```python
from build123d import *

# Parameters (mm, degrees)
ESQUISSE1_W             = 76
ESQUISSE1_H             = 76
ESQUISSE1_W_2           = 70
ESQUISSE1_H_2           = 70
BOSS_EXTRU_2_DEPTH      = 101
ESQUISSE2_W             = 76
ESQUISSE2_H             = 76
BOSS_EXTRU_3_DEPTH      = 5
ESQUISSE3_W             = 76
ESQUISSE3_H             = 76
BOSS_EXTRU_4_DEPTH      = 5
ESQUISSE4_W             = 60
ESQUISSE4_H             = 44.878799425
ESQUISSE4_H_2           = 41.121200575
ENL_V_MAT_EXTRU_1_DEPTH = 80
ESQUISSE5_W             = 43.832159463
ESQUISSE5_H             = 60
ESQUISSE5_W_2           = 42.167840537
ENL_V_MAT_EXTRU_2_DEPTH = 80
ESQUISSE8_W             = 15
ESQUISSE8_H             = 30
BOSS_EXTRU_6_DEPTH      = 50
CONG_6_R                = 10
CONG_7_R                = 10
ESQUISSE10_R            = 5.5
ENL_V_MAT_EXTRU_3_DEPTH = 25
ESQUISSE11_R            = 7.5
ENL_V_MAT_EXTRU_4_DEPTH = 1


with BuildPart() as part:
    # Esquisse1 → Boss.-Extru.2 (new body)
    with BuildSketch(Plane.XY):
        with Locations((1.043095631, -5.469290785)):
            Rectangle(ESQUISSE1_W, ESQUISSE1_H)
        with Locations((1.043095631, -5.469290785)):
            Rectangle(ESQUISSE1_W_2, ESQUISSE1_H_2, mode=Mode.SUBTRACT)
    extrude(amount=BOSS_EXTRU_2_DEPTH)

    # Esquisse2 → Boss.-Extru.3 (add)
    with BuildSketch(Plane.XY.offset(101)):
        with Locations((1.043095631, -5.469290785)):
            Rectangle(ESQUISSE2_W, ESQUISSE2_H)
    extrude(amount=BOSS_EXTRU_3_DEPTH)

    # Esquisse3 → Boss.-Extru.4 (add)
    with BuildSketch(Plane(origin=(0, 0, 0), x_dir=(-1, 0, 0), z_dir=(0, 0, -1))):
        with Locations((-1.043095631, -5.469290785)):
            Rectangle(ESQUISSE3_W, ESQUISSE3_H)
    extrude(amount=BOSS_EXTRU_4_DEPTH)

    # Esquisse4 → Enlèv. mat.-Extru.1 (cut)
    with BuildSketch(Plane(origin=(0, 32.530709215, 0), x_dir=(1, 0, 0), z_dir=(0, 1, 0))):
        with Locations((1.043095631, -27.439399713)):
            Rectangle(ESQUISSE4_W, ESQUISSE4_H)
        with Locations((1.043095631, -75.439399713)):
            Rectangle(ESQUISSE4_W, ESQUISSE4_H_2)
    extrude(amount=-ENL_V_MAT_EXTRU_1_DEPTH, mode=Mode.SUBTRACT)

    # Esquisse5 → Enlèv. mat.-Extru.2 (cut)
    with BuildSketch(Plane.ZY.offset(36.956904369)):
        with Locations((26.916079732, -5.469290785)):
            Rectangle(ESQUISSE5_W, ESQUISSE5_H)
        with Locations((74.916079732, -5.469290785)):
            Rectangle(ESQUISSE5_W_2, ESQUISSE5_H)
    extrude(amount=-ENL_V_MAT_EXTRU_2_DEPTH, mode=Mode.SUBTRACT)

    # Esquisse8 → Boss.-Extru.6 (add)
    with BuildSketch(Plane.XY.offset(106)):
        with Locations((1.043095631, -5.469290785)):
            Rectangle(ESQUISSE8_W, ESQUISSE8_H)
    extrude(amount=BOSS_EXTRU_6_DEPTH)

    # Congé6
    cong_6_edges = [part.edges().sort_by_distance(p)[0] for p in [
        (1.043095631, -20.469290785, 156),
    ]]
    fillet(cong_6_edges, radius=CONG_6_R)

    # Congé7
    cong_7_edges = [part.edges().sort_by_distance(p)[0] for p in [
        (1.043095631, 9.530709215, 156),
    ]]
    fillet(cong_7_edges, radius=CONG_7_R)

    # Esquisse10 → Enlèv. mat.-Extru.3 (cut)
    with BuildSketch(Plane.ZY.offset(6.456904369)):
        with Locations(Location((141, -5.469290785, 0), (0, 0, 270))):
            Circle(ESQUISSE10_R)
    extrude(amount=-ENL_V_MAT_EXTRU_3_DEPTH, mode=Mode.SUBTRACT)

    # Esquisse11 → Enlèv. mat.-Extru.4 (cut)
    with BuildSketch(Plane.ZY.offset(6.456904369)):
        with Locations(Location((141, -5.469290785, 0), (0, 0, 270))):
            Circle(ESQUISSE11_R)
    extrude(amount=-ENL_V_MAT_EXTRU_4_DEPTH, mode=Mode.SUBTRACT)


solid = part.part
```
Read the model definition and answer for the solid it produces. Units are mm, in the model's axes. A direction names the side the tool comes from. Coordinates: 2 decimals unless noted, no trailing zeros. Write each loop counter-clockwise with the first axis right and the second up, starting at its lowest first coordinate (ties: lowest second). Pieces come first, ordered by that corner, then holes. Notation, with made-up numbers: (20, 71.25) -> (68, 71.25) arc R23 cw to (68, 107.25) -> close; hole circle Ø10 at (-2.75, -10). An arc over 180 degrees is marked (long way). Return JSON: item names as keys, results as strings.
1. A cutting plane is placed at C-C (z = 141). Determine the outline of the cut face in (x, y), and give its area (3 significant figures).
Found:
{"outline": "(-6.46, -20.47) -> (8.54, -20.47) -> (8.54, -10.97) -> (-5.46, -10.97) -> (-5.46, -12.97) -> (-6.46, -12.97) -> close; (-6.46, 2.03) -> (-5.46, 2.03) -> (-5.46, 0.03) -> (8.54, 0.03) -> (8.54, 9.53) -> (-6.46, 9.53) -> close", "area": "281 mm2"}
2. A tool of negligible diameter and unlimited length cuts with its end or side. For faces 4 (the face through (1, 31, 5)), 5 (the face through (-35, 24.531, 27)), 6 (the face through (1, 9.531, 126)), from which of +Z, -Z, +X, -X, +Y, -Y can it reach the whole face along a straight path? Write none if from no direction.
Found:
{"face 4": "+Y, -Y", "face 5": "+X, -X", "face 6": "+Z, +X, -X, +Y"}
3. Each of these flat-tipped pins is pushed along its axis until it touches: P1, Ø0.9, axis at x = 12.5, y = 31, coming from the +Z side; P2, Ø4.5, axis at x = 1.5, z = 128.5, coming from the +Y side; P3, Ø4, axis at y = -24, z = 113, coming from the -X side; P4, Ø10, axis at y = -11, z = 58.5, coming from the -X side. Where does it stop, or does it pass through?
Found:
{"P1": "z = 106", "P2": "y = 9.53", "P3": "through", "P4": "x = -36.96"}
4. A cutting plane is placed at B-B (y = -30). Determine the outline of the cut face in (x, z).
Found:
{"outline": "(-36.96, -5) -> (39.04, -5) -> (39.04, 5) -> (36.04, 5) -> (36.04, 0) -> (-33.96, 0) -> (-33.96, 5) -> (-36.96, 5) -> close; (-36.96, 48.83) -> (-33.96, 48.83) -> (-33.96, 53.83) -> (-36.96, 53.83) -> close; (-36.96, 96) -> (-33.96, 96) -> (-33.96, 101) -> (36.04, 101) -> (36.04, 96) -> (39.04, 96) -> (39.04, 106) -> (-36.96, 106) -> close; (36.04, 48.83) -> (39.04, 48.83) -> (39.04, 53.83) -> (36.04, 53.83) -> close"}
5. A cutting plane is placed at D-D (z = 124). Determine the outline of the cut face in (x, y), and give its area (3 significant figures).
Found:
{"outline": "(-6.46, -20.47) -> (8.54, -20.47) -> (8.54, 9.53) -> (-6.46, 9.53) -> close", "area": "450 mm2"}
6. A cutting plane is placed at A-A (x = 25.5). Determine the outline of the cut face in (y, z).
Found:
{"outline": "(-43.47, -5) -> (32.53, -5) -> (32.53, 5) -> (29.53, 5) -> (29.53, 0) -> (-40.47, 0) -> (-40.47, 5) -> (-43.47, 5) -> close; (-43.47, 49.88) -> (-40.47, 49.88) -> (-40.47, 54.88) -> (-43.47, 54.88) -> close; (-43.47, 96) -> (-40.47, 96) -> (-40.47, 101) -> (29.53, 101) -> (29.53, 96) -> (32.53, 96) -> (32.53, 106) -> (-43.47, 106) -> close; (29.53, 49.88) -> (32.53, 49.88) -> (32.53, 54.88) -> (29.53, 54.88) -> close"}
7. Determine the mould class of faces 1 (the face through (1, -42, 54.879)), 2 (the face through (-35, -35.469, 27)), 3 (the face through (31.043, -42, 76)) for opening direction X: pulls with the +X half, pulls with the -X half, needs draft (parallel to the pull), parting line crosses it, or undercut.
Found:
{"face 1": "undercut", "face 2": "needs draft", "face 3": "undercut"}
8. Find the intervals of material crossed by line 1 along Z through (x, y) = (10, -11); line 2 along Y through (x, z) = (-19, 53); line 3 along X through (y, z) = (27, 18), in increasing order. Write a range as from..to.
Found:
{"line 1": "-5..0, 101..106", "line 2": "-43.47..-40.47, 29.53..32.53", "line 3": "-36.96..-33.96, 36.04..39.04"}
